The listing builds one solid part. Answer for the finished solid, in the listing's coordinates (mm). A direction names the side the tool comes from. Round coordinates to 2 decimals unless told otherwise and drop trailing zeros. Write each loop counter-clockwise with the first axis right and the second up, starting at its lowest first coordinate (ties: lowest second). Pieces come first, ordered by that corner, then holes. Notation, with made-up numbers: (48.25, 27.25) - (58.25, 27.25) arc R26 ccw to (58.25, 48.25) - close; hole circle Ø1 at (26.25, -31). An arc over 180 degrees is marked (long way). Return JSON: item names as keys, results as strings. Group by question number.
(1) Section D-D, the plane y = -0.57 is taken. Write down the section's boundary in (x, z).
(2) Each of these flat-tipped pins is pushed along its axis until it touches: pin 1 (6 mm diameter, centred on x = -2.5, y = -0.5, fed in from +Z); pin 2 (1.7 mm diameter, centred on x = -2, y = -14, fed in from -Z); pin 3 (1.8 mm diameter, centred on x = 0, z = -35.5, fed in from -Y). Where does it stop, or does it pass through?
(3) Section C-C, the plane x = 3 is taken. Write down the section's boundary in (y, z), then the cut area to 3 significant figures.
(4) Find the intervals of material crossed by line 1 along Y through (x, z) = (-4.75, -31); line 2 along X through (y, z) = (-14, -32); line 3 along Y through (x, z) = (-2, -35.6), in increasing order. Write a range as [from, to].
(5) Determine the mould class of faces 6 (the flat face through (5, 0, -33)), 7 (the flat face through (-2, -12, -30)), 8 (the flat face through (-9, 0, -33)), 9 (the cylindrical face through (-2.235, 11.926, -34.726)) for opening direction X: +X half, -X half, draft (parallel to the pull), parting line (faces both ways), or undercut.
(6) Section A-A, the plane y = -14 is taken. Write down the section's boundary in (x, z), then the cut area to 4 significant figures.
(7) Section B-B, the plane z = -28.5 is taken. Write down the section's boundary in (x, y).
(8) Which of the six approach directions +Z, -Z, +X, -X, +Y, -Y give full straight-line access (tool end or side, diameter ignored) to faces 1 (the flat face through (-2, -17, -30)), 2 (the flat face through (-2, 4, -33)), 3 (the flat face through (-2, 12, -30)), 4 (the flat face through (-2, -5.3, -35)), 5 (the flat face through (-2, 13, -35))?
```python
from build123d import *

# Parameters (mm, degrees)
CYLINDER001_R          = 3.5
CYLINDER001_DEPTH      = 4
CYLINDER001_ROLL_ANGLE = 90
CYLINDER003_R          = 0.65
CYLINDER003_DEPTH      = 6
CYLINDER003_ROLL_ANGLE = 90
CYLINDER_R             = 6.5
CYLINDER_DEPTH         = 4
CYLINDER_ROLL_ANGLE    = 90
CYLINDER002_R          = 0.65
CYLINDER002_DEPTH      = 6
CYLINDER002_ROLL_ANGLE = 90
PAD002_DEPTH           = 7
CUT003_ROLL_ANGLE      = 90
CUT003_PLACEMENT_ANGLE = -90


with BuildPart() as cylinder001:
    # Cylinder001 → Cylinder001 (new body)
    with BuildSketch(Plane.XY):
        Circle(CYLINDER001_R)
    extrude(amount=CYLINDER001_DEPTH)


with BuildPart() as cylinder001_1:
    # Cylinder001 roll: moved
    add(cylinder001.part.rotate(Axis((0, 0, 0), (1, 0, 0)), CYLINDER001_ROLL_ANGLE))


with BuildPart() as cylinder001_2:
    # Cylinder001 placement: moved
    add(cylinder001_1.part.moved(Location((0.57, -7, 0))))


with BuildPart() as cylinder003:
    # Cylinder003 → Cylinder003 (new body)
    with BuildSketch(Plane.XY):
        Circle(CYLINDER003_R)
    extrude(amount=CYLINDER003_DEPTH)


with BuildPart() as cylinder003_1:
    # Cylinder003 roll: moved
    add(cylinder003.part.rotate(Axis((0, 0, 0), (1, 0, 0)), CYLINDER003_ROLL_ANGLE))


with BuildPart() as cylinder003_2:
    # Cylinder003 placement: moved
    add(cylinder003_1.part.moved(Location((14, -1, 0))))


with BuildPart() as cylinder:
    # Cylinder → Cylinder (new body)
    with BuildSketch(Plane.XY):
        Circle(CYLINDER_R)
    extrude(amount=CYLINDER_DEPTH)


with BuildPart() as cylinder_1:
    # Cylinder roll: moved
    add(cylinder.part.rotate(Axis((0, 0, 0), (1, 0, 0)), CYLINDER_ROLL_ANGLE))


with BuildPart() as cylinder_2:
    # Cylinder placement: moved
    add(cylinder_1.part.moved(Location((-5.43, -7, 0))))


with BuildPart() as fusion001:
    # Cylinder002 → Cylinder002 (new body)
    with BuildSketch(Plane.XY):
        Circle(CYLINDER002_R)
    extrude(amount=CYLINDER002_DEPTH)


with BuildPart() as fusion001_1:
    # Cylinder002 roll: moved
    add(fusion001.part.rotate(Axis((0, 0, 0), (1, 0, 0)), CYLINDER002_ROLL_ANGLE))


with BuildPart() as fusion001_2:
    # Cylinder002 placement: moved
    add(fusion001_1.part.moved(Location((-14, -1, 0))))

    # Fusion001: union Cylinder001, Cylinder003, Cylinder
    add(cylinder001_2.part)
    add(cylinder003_2.part)
    add(cylinder_2.part)


with BuildPart() as cut003:
    # Sketch → Pad002 (new body, symmetric)
    with BuildSketch(Plane.XY):
        Polygon((-17, -1.5), (-12, -1.5), (-12, -6.3), (12, -6.3), (12, -1.5), (17, -1.5), (17, -7), (5.3, -7), (5.3, -10.5), (-13, -10.5), (-13, -7), (-17, -7), align=None)
    extrude(amount=PAD002_DEPTH, both=True)

    # Cut003: cut Fusion001
    add(fusion001_2.part, mode=Mode.SUBTRACT)


with BuildPart() as cut003_1:
    # Cut003 roll: moved
    add(cut003.part.rotate(Axis((0, 0, 0), (1, 0, 0)), CUT003_ROLL_ANGLE))


with BuildPart() as cut003_2:
    # Cut003 placement: moved
    add(cut003_1.part.moved(Location((-2, 0, -26))).rotate(Axis((-2, 0, -26), (0, 0, 1)), CUT003_PLACEMENT_ANGLE))


solid = cut003_2.part
```
Working result:
{
 "1": {"outline": "(-9, -36.5) - (-5.5, -36.5) - (-5.5, -33) - (1.5, -33) - (1.5, -36.5) - (5, -36.5) - (5, -32.3) - (-9, -32.3) - close"},
 "2": {"pin 1": "stops at z = -32.3", "pin 2": "stops at z = -33", "pin 3": "stops at y = -5.3"},
 "3": {"outline": "(-17, -33) - (-5.3, -33) - (-5.3, -36.5) - (1.28, -36.5) - (1.28, -33) - (9.58, -33) - (9.58, -36.5) - (13, -36.5) - (13, -33) - (17, -33) - (17, -27.5) - (12, -27.5) - (12, -32.3) - (-12, -32.3) - (-12, -27.5) - (-17, -27.5) - close", "area": "107 mm^2"},
 "4": {"line 1": "y = [-17, -12], [12, 17]", "line 2": "x = [-9, -2.65], [-1.35, 5]", "line 3": "y = [-5.3, -4.07], [11.93, 13]"},
 "5": {"face 6": "+X half", "face 7": "draft", "face 8": "-X half", "face 9": "undercut"},
 "6": {"outline": "(-9, -33) - (-2.65, -33) - (-2.65, -27.5) - (-9, -27.5) - close; (-1.35, -33) - (5, -33) - (5, -27.5) - (-1.35, -27.5) - close", "area": "69.85 mm^2"},
 "7": {"outline": "(-9, -17) - (5, -17) - (5, -12) - (-9, -12) - close; (-9, 12) - (5, 12) - (5, 17) - (-9, 17) - close; hole circle Ø1.3 at (-2, -14); hole circle Ø1.3 at (-2, 14)"},
 "8": {"face 1": "+Z, -Z, +X, -X, -Y", "face 2": "-Z", "face 3": "+Z, +X, -X", "face 4": "-Z, +X, -X, -Y", "face 5": "-Z, +X, -X, +Y"}
}
